The model under review builds one solid part; all positions refer to its coordinate system, in mm. A direction names the side the tool comes from. Round coordinates to 2 decimals unless told otherwise and drop trailing zeros. Loops run counter-clockwise (first coordinate to the right, second up) from the corner with the lowest first, then second, coordinate; pieces in that order, holes last. Notation, with made-up numbers: (44, 28.5) -> (98, 28.5) arc R18 ccw to (98, 55.5) -> close; hole circle Ø5 at (23, 89). An arc over 180 degrees is marked (long way). Use a Markdown table: item, result. Add a question column.
1) Consider section C-C on y = 33. Give the boundary of the cut face in (x, z).
2) Consider section A-A on z = 0. Give the boundary of the cut face in (x, y), plus the area to 3 significant figures.
3) Consider section B-B on x = 0. Give the boundary of the cut face in (y, z), plus the area to 3 significant figures.
4) Mouldability with a two-part tool opening along X and no side actions: class faces 1 (the flat face through (12, 41, -8)), 2 (the flat face through (10, 28, 0)), 3 (the flat face through (33, 5, 14)) as released by +X, released by -X, zero draft, split by the parting line, or undercut.
5) For faces 4 (the flat face through (9, 2, -20)), 5 (the flat face through (0, 32, -13)), 6 (the flat face through (0, 10, 18)), 7 (the flat face through (23, 12, -11)), 8 (the flat face through (-23, 12, -11)), list the 3-axis set-ups (+Z, -Z, +X, -X, +Y, -Y) from which the entire face can be reached by the end or side of a thin tool; tool diameter is ignored.
6) Insertion check: pin 1 (19 mm diameter, centred on x = -2, z = 6.5, fed in from -Y); pin 2 (5 mm diameter, centred on x = -0.5, z = 6, fed in from +Y) (3 decimals); pin 3 (4 mm diameter, centred on x = -12, y = 23.5, fed in from +Z); pin 4 (10 mm diameter, centred on x = -22.5, z = 2, fed in from +Y). Each pin has a flat end and moves straight along its axis. Give the tip position at first contact, or say it passes through.
7) Wall thickness on probe 1 along X at (y, z) = (2, 0); probe 2 along Z at (x, y) = (30, 8.5); probe 3 along Y at (x, z) = (0, 12.5): over which ranges is each line inside the solid? List them lowest first.
8) Consider section D-D on y = 9. Give the boundary of the cut face in (x, z).
from build123d import *

# Parameters (mm, degrees)
SKETCH_1_W          = 66
SKETCH_1_H          = 46
EXTRUDE_1_DEPTH     = 10
SKETCH_2_W          = 66
SKETCH_2_H          = 22
EXTRUDE_2_DEPTH     = 4
SKETCH_3_R          = 17
EXTRUDE_3_DEPTH     = 50
SKETCH_4_W          = 18
SKETCH_4_H          = 4
CUT_EXTRUDE_1_DEPTH = 47
CUT_EXTRUDE_2_DEPTH = 15
SKETCH_6_W          = 20
SKETCH_6_H          = 20
CUT_EXTRUDE_3_DEPTH = 51
CUT_EXTRUDE_4_DEPTH = 18
SKETCH_8_R          = 7
CUT_EXTRUDE_5_DEPTH = 24
SKETCH_9_R          = 19
CUT_EXTRUDE_6_DEPTH = 6


with BuildPart() as part:
    # 草图1 → 凸台-拉伸1 (new body)
    with BuildSketch(Plane(origin=(0, 0, 0), x_dir=(1, 0, 0), z_dir=(0, 1, 0))):
        Rectangle(SKETCH_1_W, SKETCH_1_H)
    extrude(amount=EXTRUDE_1_DEPTH)

    # 草图2 → 凸台-拉伸2 (add)
    with BuildSketch(Plane(origin=(0, 10, 0), x_dir=(1, 0, 0), z_dir=(0, 1, 0))):
        Rectangle(SKETCH_2_W, SKETCH_2_H)
    extrude(amount=EXTRUDE_2_DEPTH)

    # 草图3 → 凸台-拉伸3 (add)
    with BuildSketch(Plane(origin=(0, 0, 0), x_dir=(1, 0, 0), z_dir=(0, 1, 0))):
        Circle(SKETCH_3_R)
    extrude(amount=EXTRUDE_3_DEPTH)

    # 草图4 → 切除-拉伸1 (cut, through all)
    with BuildSketch(Plane.XY.offset(23)):
        with Locations((0, 2)):
            Rectangle(SKETCH_4_W, SKETCH_4_H)
    extrude(amount=-CUT_EXTRUDE_1_DEPTH, mode=Mode.SUBTRACT)

    # 草图5 → 切除-拉伸2 (cut, through all)
    with BuildSketch(Plane(origin=(0, 14, 0), x_dir=(1, 0, 0), z_dir=(0, 1, 0))):
        with BuildLine():
            Line((-28, 5), (-33, 5))
            Line((-33, 5), (-33, -5))
            Line((-33, -5), (-28.383132006, -4.985299376))
            ThreePointArc((-28.383132006, -4.985299376), (-23.003676508, -0.191706965), (-28, 5))
        make_face()
        with BuildLine():
            Line((33, -5), (28.383132006, -4.985299376))
            ThreePointArc((28.383132006, -4.985299376), (23.003676508, -0.191706965), (28, 5))
            Line((28, 5), (33, 5))
            Line((33, 5), (33, -5))
        make_face()
    extrude(amount=-CUT_EXTRUDE_2_DEPTH, mode=Mode.SUBTRACT)

    # 草图6 → 切除-拉伸3 (cut, through all)
    with BuildSketch(Plane(origin=(0, 50, 0), x_dir=(1, 0, 0), z_dir=(0, 1, 0))):
        Rectangle(SKETCH_6_W, SKETCH_6_H)
    extrude(amount=-CUT_EXTRUDE_3_DEPTH, mode=Mode.SUBTRACT)

    # 草图7 → 切除-拉伸4 (cut)
    with BuildSketch(Plane(origin=(0, 50, 0), x_dir=(1, 0, 0), z_dir=(0, 1, 0))):
        with BuildLine():
            Line((-15, 8), (-10, 8))
            Line((-10, 8), (-10, 10))
            Line((-10, 10), (10, 10))
            Line((10, 10), (10, 8))
            Line((10, 8), (15, 8))
            ThreePointArc((15, 8), (0, 17), (-15, 8))
        make_face()
    extrude(amount=-CUT_EXTRUDE_4_DEPTH, mode=Mode.SUBTRACT)

    # 草图8 → 切除-拉伸5 (cut, through all)
    with BuildSketch(Plane.XY):
        with Locations((0, 32)):
            Circle(SKETCH_8_R)
    extrude(amount=CUT_EXTRUDE_5_DEPTH, mode=Mode.SUBTRACT)

    # 草图9 → 切除-拉伸6 (cut)
    with BuildSketch(Plane(origin=(0, 0, 0), x_dir=(1, 0, 0), z_dir=(0, 1, 0))):
        Circle(SKETCH_9_R)
    extrude(amount=CUT_EXTRUDE_6_DEPTH, mode=Mode.SUBTRACT)


solid = part.part
Result set:
| question | item | result |
|---|---|---|
| 1 | outline | (-15, -8) -> (-10, -8) -> (-10, 10) -> (-6.93, 10) -> (-6.93, 15.52) arc R17 ccw to start; (6.93, 10) -> (10, 10) -> (10, -8) -> (15, -8) arc R17 ccw to (6.93, 15.52) -> close |
| 2 | outline | (-23, 0) -> (-19, 0) -> (-19, 6) -> (-10, 6) -> (-10, 50) -> (-17, 50) -> (-17, 14) -> (-23, 14) -> close; (10, 6) -> (19, 6) -> (19, 0) -> (23, 0) -> (23, 14) -> (17, 14) -> (17, 50) -> (10, 50) -> close |
| 2 | area | 760 mm2 |
| 3 | outline | (4, -23) -> (10, -23) -> (10, -17) -> (32, -17) -> (32, -10) -> (6, -10) -> (6, -19) -> (4, -19) -> close; (4, 19) -> (6, 19) -> (6, 10) -> (25, 10) -> (25, 17) -> (10, 17) -> (10, 23) -> (4, 23) -> close; (39, 10) -> (50, 10) -> (50, 17) -> (39, 17) -> close |
| 3 | area | 456 mm2 |
| 4 | face 1 | zero draft |
| 4 | face 2 | undercut |
| 4 | face 3 | released by +X |
| 5 | face 4 | +Z, -Z, -Y |
| 5 | face 5 | -Z, +X, -X, +Y |
| 5 | face 6 | +Z, +Y |
| 5 | face 7 | -Z, +X, +Y |
| 5 | face 8 | -Z, -X, +Y |
| 6 | pin 1 | y = 6 |
| 6 | pin 2 | through |
| 6 | pin 3 | z = 13.75 |
| 6 | pin 4 | y = 14 |
| 7 | probe 1 | -23 to -19, 19 to 23 |
| 7 | probe 2 | -23 to -5, 4.99 to 23 |
| 7 | probe 3 | 6 to 25, 39 to 50 |
| 8 | outline | (-33, -23) -> (33, -23) -> (33, -5) -> (28, -5) arc R5 cw (long way) to (28.38, 4.99) -> (33, 5) -> (33, 23) -> (-33, 23) -> (-33, 5) -> (-28.38, 4.99) arc R5 cw (long way) to (-28, -5) -> (-33, -5) -> close; hole (-10, -10) -> (10, -10) -> (10, 10) -> (-10, 10) -> close |
